Could you check a few things on this drawing? It's one solid part, dimensions in mm from its lowest x, y, z. Give positions to 0.01 mm unless a question says otherwise; leave off trailing zeros. Loops run counter-clockwise (first coordinate to the right, second up) from the corner with the lowest first, then second, coordinate; pieces in that order, holes last. Notation, with made-up numbers: M -16.5,20 L 15.5,20 A34 cw 15.5,57 Z; hole C 30,57 d4. An arc over 180 degrees is marked long. One line per item, written item: value. Start each with the question number.
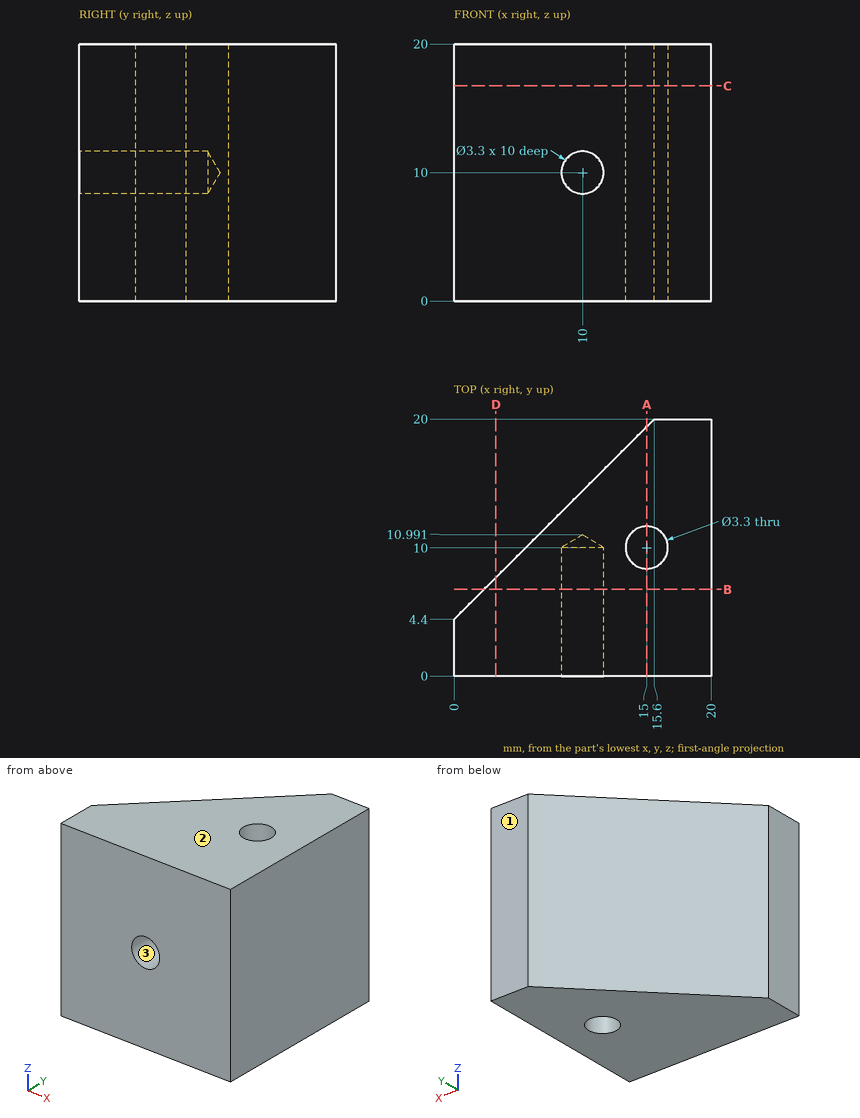
Q1. If we section it at D-D, the plane x = 3.25: Write out the boundary of the cut face in (y, z).
Q2. For P1, Ø6, axis at y = 14, z = 8.5, coming from the -X side; P2, Ø1.5, axis at x = 14.5, z = 14.5, coming from the +Y side; P3, Ø2.5, axis at x = 15, y = 10, coming from the +Z side; P4, Ø2.5, axis at x = 10, z = 10, coming from the +Y side, each with a flat end and sliding along its axis, tell me the tip position at first contact or that it passes through.
Q3. If we section it at A-A, the plane x = 15: Write out the boundary of the cut face in (y, z).
Q4. If we mould it in two halves opening along Z, with no side actions, what happens to the marked faces 1, 2 and 3? For each: released by +Z, released by -Z, zero draft, split by the parting line, or undercut.
Q5. I need wall thicknesses on line 1 along Z through (x, y) = (10, 5.5); line 2 along Y through (x, z) = (7.25, 4.5); line 3 along Y through (x, z) = (16.25, 10.5) (1 decimal). Which ranges of each line are inside material? Lowest first, please.
Q6. If we section it at B-B, the plane y = 6.75: Write out the boundary of the cut face in (x, z).
Q7. If we section it at C-C, the plane z = 16.75: Write out the boundary of the cut face in (x, y), plus the area to 3 significant figures.
Response:
1. outline: M 0,0 L 7.65,0 L 7.65,20 L 0,20 Z
2. P1: x = 6.6
2. P2: y = 19.65
2. P3: through
2. P4: y = 15.65
3. outline: M 0,0 L 8.35,0 L 8.35,20 L 0,20 Z; M 11.65,0 L 19.4,0 L 19.4,20 L 11.65,20 Z
4. face 1: zero draft
4. face 2: released by +Z
4. face 3: undercut
5. line 1: 0 to 8.35, 11.65 to 20
5. line 2: 0 to 11.65
5. line 3: 0 to 8.9, 11.1 to 20
6. outline: M 2.35,0 L 20,0 L 20,20 L 2.35,20 Z; hole C 10,10 d3.3
7. outline: M 0,0 L 20,0 L 20,20 L 15.6,20 L 0,4.4 Z; hole C 15,10 d3.3
7. area: 270 mm^2
